```python
from build123d import *

# Parameters (mm, degrees)
SKETCH1_W           = 10
SKETCH1_H           = 40
BOSS_EXTRUDE3_DEPTH = 40
SKETCH1_5_W         = 15
SKETCH1_5_H         = 40
BOSS_EXTRUDE4_DEPTH = 30
SKETCH1_6_W         = 15
SKETCH1_6_H         = 40
BOSS_EXTRUDE5_DEPTH = 15


with BuildPart() as part:
    # Sketch1 → Boss-Extrude3 (new body)
    with BuildSketch(Plane.XY):
        with Locations((-35, 20)):
            Rectangle(SKETCH1_W, SKETCH1_H)
    extrude(amount=BOSS_EXTRUDE3_DEPTH)

    # Sketch1<5> → Boss-Extrude4 (add)
    with BuildSketch(Plane.XY):
        with Locations((-22.5, 20)):
            Rectangle(SKETCH1_5_W, SKETCH1_5_H)
    extrude(amount=BOSS_EXTRUDE4_DEPTH)

    # Sketch1<6> → Boss-Extrude5 (add)
    with BuildSketch(Plane.XY):
        with Locations((-7.5, 20)):
            Rectangle(SKETCH1_6_W, SKETCH1_6_H)
    extrude(amount=BOSS_EXTRUDE5_DEPTH)


solid = part.part
```
Source: CAD feature listing. Evaluate the final solid. Frame: model axes, mm. A direction names the side the tool comes from. Coordinates: 2 decimals unless noted, no trailing zeros. Loops run counter-clockwise (first coordinate to the right, second up) from the corner with the lowest first, then second, coordinate; pieces in that order, holes last. Notation, with made-up numbers: M -1,88 L 47,88 A11 cw 47,100 Z; hole C -7.5,51.25 d4. An arc over 180 degrees is marked long. Use a Markdown table: item, result. Add a question column.
Q1. Section query A-A, the plane y = 3. Return loops of the section in (x, z).
Q2. Material intervals for L1, parallel to X at y = 9.5, z = 19; L2, parallel to Z at x = -5.5, y = 17; L3, parallel to X at y = 16, z = 35, sorted ascending.
Q3. Section query B-B, the plane z = 16.5. Return loops of the section in (x, y).
Q4. First-contact query: pin 1 (16.5 mm diameter, centred on x = -5, y = 11.5, fed in from +Z); pin 2 (1.5 mm diameter, centred on y = 32.5, z = 19, fed in from +X); pin 3 (1.5 mm diameter, centred on x = -18, y = 24.5, fed in from +Z). Flat tips, straight axial feed; report the tip coordinate or a pass-through.
Q5. Section query C-C, the plane x = -24.5. Return loops of the section in (y, z), and give its area (3 significant figures).
Q6. Access query for faces 1 (the flat face through (-15, 20, 22)), 2 (the flat face through (-25, 0, 15)). Directions: +Z, -Z, +X, -X, +Y, -Y. A direction counts if a zero-diameter tool reaches every point of the face in a straight line with its end or side. Return the directions, or none.
Result:
| question | item | result |
|---|---|---|
| 1 | outline | M -40,0 L 0,0 L 0,15 L -15,15 L -15,30 L -30,30 L -30,40 L -40,40 Z |
| 2 | L1 | x = -40 to -15 |
| 2 | L2 | z = 0 to 15 |
| 2 | L3 | x = -40 to -30 |
| 3 | outline | M -40,0 L -15,0 L -15,40 L -40,40 Z |
| 4 | pin 1 | stops at z = 15 |
| 4 | pin 2 | stops at x = -15 |
| 4 | pin 3 | stops at z = 30 |
| 5 | outline | M 0,0 L 40,0 L 40,30 L 0,30 Z |
| 5 | area | 1,200 mm2 |
| 6 | face 1 | +Z, +X, +Y, -Y |
| 6 | face 2 | +Z, -Z, +X, -X, -Y |
